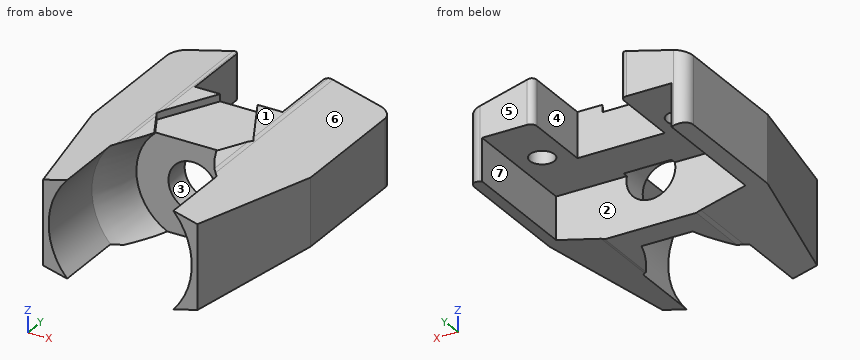
from build123d import *

# Parameters (mm, degrees)
PAD_DEPTH       = 12
POCKET_DEPTH    = 62
SKETCH019_W     = 31
SKETCH019_H     = 21.780884
POCKET002_DEPTH = 17
SKETCH020_R     = 2
POCKET003_DEPTH = 4
CYLINDER_R      = 4
CYLINDER_DEPTH  = 28
POCKET032_DEPTH = 5
SKETCH084_W     = 7.885986
SKETCH084_H     = 7.189331
PAD020_DEPTH    = 0.5


with BuildPart() as part:
    # Sketch010 → Pad (new body, symmetric)
    with BuildSketch(Plane.XY):
        with BuildLine():
            Line((12.639868, 59.984547), (-12.639868, 59.984547))
            Line((-12.639868, 59.984547), (-17.867889, 82.058411))
            Line((-17.867889, 82.058411), (-17.867889, 102.222236))
            ThreePointArc((-15.867889, 104.222236), (-17.282103, 103.63645), (-17.867889, 102.222236))
            Line((-15.867889, 104.222236), (-8.154342, 104.222236))
            ThreePointArc((-7.154342, 103.222236), (-7.447235, 103.929343), (-8.154342, 104.222236))
            Line((-7.154342, 103.222236), (-7.154342, 92.189331))
            Line((-7.154342, 92.189331), (7.154342, 92.189331))
            Line((7.154342, 92.189331), (7.154342, 103.222236))
            ThreePointArc((8.154342, 104.222236), (7.447235, 103.929343), (7.154342, 103.222236))
            Line((8.154342, 104.222236), (15.867889, 104.222236))
            ThreePointArc((17.867889, 102.222236), (17.282103, 103.63645), (15.867889, 104.222236))
            Line((17.867889, 102.222236), (17.867889, 82.058411))
            Line((17.867889, 82.058411), (12.639868, 59.984547))
        make_face()
    extrude(amount=PAD_DEPTH, both=True)

    # Sketch011 → Pocket (cut)
    with BuildSketch(Plane.XZ.offset(-54)):
        Polygon((0, 13.813917), (-22.117895, 13.813917), (-22.117895, -0.189388), (-22.117895, -17.743416), (0, -17.743416), (22.658901, -17.743416), (22.658901, -0.111897), (22.658901, 13.813917), align=None)
        Polygon((-18.596464, 0), (-18.596464, 5.287208), (-8.154342, 8), (-7.443202, 8.179805), (0, 8.179805), (7.519913, 8.179805), (8.154342, 8), (18.531284, 5.287208), (18.531284, -0.112287), (18.531284, -5.399495), (8.154342, -8), (7.554242, -8.253323), (0.11104, -8.253323), (-7.443202, -8.253323), (-8.154342, -8), (-18.596464, -5.371119), align=None, mode=Mode.SUBTRACT)
    extrude(amount=-POCKET_DEPTH, mode=Mode.SUBTRACT)

    # Sketch019 → Pocket002 (cut)
    with BuildSketch(Plane.XY.offset(0.8)):
        with Locations((0.01352, 95.005211)):
            Rectangle(SKETCH019_W, SKETCH019_H)
    extrude(amount=-POCKET002_DEPTH, mode=Mode.SUBTRACT)

    # Sketch020 → Pocket003 (cut)
    with BuildSketch(Plane.XY.offset(0.8)):
        with Locations((-11.1, 94.9)):
            Circle(SKETCH020_R)
        with Locations((11.3, 94.9)):
            Circle(SKETCH020_R)
        with Locations((0.013518, 88.3)):
            Circle(SKETCH020_R)
    extrude(amount=POCKET003_DEPTH, mode=Mode.SUBTRACT)

    # Cylinder → Cylinder (cut)
    with BuildSketch(Plane.XZ.offset(-85)):
        Circle(CYLINDER_R)
    extrude(amount=CYLINDER_DEPTH, mode=Mode.SUBTRACT)

    # Sketch067 → Pocket032 (cut)
    with BuildSketch(Plane.XY.offset(7)):
        Polygon((-7.9, 83), (0, 68), (7.9, 83), (0, 98), align=None)
    extrude(amount=POCKET032_DEPTH, mode=Mode.SUBTRACT)

    # Sketch084 → Pad020 (join)
    with BuildSketch(Plane.XY.offset(0.8)):
        with Locations((-0.023809, 88.594665)):
            Rectangle(SKETCH084_W, SKETCH084_H)
    extrude(amount=PAD020_DEPTH)

    # Sketch085 → Groove (revolve, cut)
    with BuildSketch(Plane.XY):
        with BuildLine():
            ThreePointArc((9.252061, 79.708405), (10.164814, 75.624968), (11.720768, 71.740822))
            Line((11.720768, 71.740822), (11.720768, 58.4589))
            Line((11.720768, 58.4589), (0, 58.4589))
            Line((0, 58.4589), (0, 79.708405))
            Line((9.252061, 79.708405), (0, 79.708405))
        make_face()
    revolve(axis=Axis((0, 0, 0), (0, 1, 0)), mode=Mode.SUBTRACT)


solid = part.part
For this review, take the finished solid that the model builds, in its own axes (mm). Face numbers are marked on the shaded views. A direction names the side the tool comes from. Give positions to 0.01 mm unless a question says otherwise; leave off trailing zeros. Order: outer loops, then holes, each group sorted by start corner. A loop starts at its lowest first (then second) coordinate and runs counter-clockwise, first axis right, second up. Notation, with made-up numbers: M 76,86.25 L 134,86.25 A8 ccw 134,94.25 Z; hole C -28,84.5 d2. An arc over 180 degrees is marked long. Answer in a Markdown table with one row per item. Add a question column.
(1) Mouldability with a two-part tool opening along X and no side actions: class the marked faces 5, 6 and 7 as +X half, -X half, draft (parallel to the pull), parting line (faces both ways), or undercut.
(2) For pin 1 (6 mm diameter, centred on x = -3, z = 3.5, fed in from -Y); pin 2 (2 mm diameter, centred on x = 0, y = 88, fed in from +Z); pin 3 (3 mm diameter, centred on x = -12, y = 95.5, fed in from -Z); pin 4 (6 mm diameter, centred on x = -2, y = 98, fed in from -Z), all flat-tipped, find the tip position at first contact; note any pin that passes through.
(3) Consider section C-C on y = 88.3. State the section outline as (x, z) points.
(4) Consider section B-B on x = 0. State the section outline as (y, z) points, and give its area (3 significant figures).
(5) Consider section D-D on y = 70.5. State the section outline as (x, z) points.
(6) For the marked faces 1, 2, 3 and 4, list the 3-axis set-ups (+Z, -Z, +X, -X, +Y, -Y) from which the entire face can be reached by the end or side of a thin tool; tool diameter is ignored.
(7) Wall thickness on probe 1 along Z at (x, y) = (0, 83.9); probe 2 along X at (y, z) = (86.5, -4); probe 3 along X at (y, z) = (83, 0): over which ranges is each line inside the solid? List them lowest first. Write a range as [from, to].
(8) Consider section A-A on y = 97.5. State the section outline as (x, z) points.
Evaluation:
| question | item | result |
|---|---|---|
| 1 | face 5 | draft |
| 1 | face 6 | +X half |
| 1 | face 7 | undercut |
| 2 | pin 1 | stops at y = 79.71 |
| 2 | pin 2 | stops at z = 7 |
| 2 | pin 3 | stops at z = 0.8 |
| 2 | pin 4 | passes through |
| 3 | outline | M -17.87,-5.55 L -15.49,-6.15 L -15.49,0.8 L 15.51,0.8 L 15.51,-6.16 L 17.87,-5.57 L 17.87,5.46 L 8.15,8 L 7.52,8.18 L 5.11,8.18 L 5.11,7 L -5.11,7 L -5.11,8.18 L -7.44,8.18 L -8.15,8 L -17.87,5.48 Z; hole M -1.99,1.3 L 2.01,1.3 L 2.01,4.8 L -1.99,4.8 Z |
| 4 | outline | M 79.71,-8.25 L 84.11,-8.25 L 84.11,-4 L 79.71,-4 Z; M 79.71,4 L 85,4 L 85,0.8 L 92.19,0.8 L 92.19,7 L 79.71,7 Z; hole M 86.3,1.3 L 90.3,1.3 L 90.3,4.8 L 86.3,4.8 Z |
| 4 | area | 65.2 mm^2 |
| 5 | outline | M -15.13,-6.24 L -8.69,-7.87 A11.72 cw -8.7,7.86 L -15.13,6.19 Z; M 8.69,-7.87 L 15.13,-6.25 L 15.13,6.18 L 8.7,7.86 A11.72 cw Z |
| 6 | face 1 | +Z, +X, -X, +Y, -Y |
| 6 | face 2 | -Z, +Y |
| 6 | face 3 | -Y |
| 6 | face 4 | +Z, -Z, +Y |
| 7 | probe 1 | z = [-8.25, -4], [4, 7] |
| 7 | probe 2 | x = [-17.87, -15.49], [15.51, 17.87] |
| 7 | probe 3 | x = [-17.87, -4], [4, 17.87] |
| 8 | outline | M -17.87,-5.55 L -15.49,-6.15 L -15.49,0.8 L -7.15,0.8 L -7.15,8.18 L -7.44,8.18 L -8.15,8 L -17.87,5.48 Z; M 7.15,0.8 L 15.51,0.8 L 15.51,-6.16 L 17.87,-5.57 L 17.87,5.46 L 8.15,8 L 7.52,8.18 L 7.15,8.18 Z |
